```python
from build123d import *

# Parameters (mm, degrees)
SKETCH1_R           = 5
SKETCH1_R_2         = 1
BOSS_EXTRUDE1_DEPTH = 3
SKETCH2_R           = 8
BOSS_EXTRUDE2_DEPTH = 4
SKETCH4_R           = 1
CUT_EXTRUDE2_DEPTH  = 8
SKETCH3_RX          = 5.25
SKETCH3_RY          = 3.5
CUT_EXTRUDE1_DEPTH  = 2
SKETCH10_R          = 1
CUT_EXTRUDE5_DEPTH  = 7
SKETCH9_R           = 1.55
CUT_EXTRUDE4_DEPTH  = 3.5
CUT_EXTRUDE9_DEPTH  = 10
FILLET3_R           = 1
FILLET1_R           = 0.4


with BuildPart() as part:
    # Sketch1 → Boss-Extrude1 (new body)
    with BuildSketch(Plane.XY):
        Circle(SKETCH1_R)
        Circle(SKETCH1_R_2, mode=Mode.SUBTRACT)
    extrude(amount=BOSS_EXTRUDE1_DEPTH)

    # Sketch2 → Boss-Extrude2 (add)
    with BuildSketch(Plane.XY.offset(3)):
        Circle(SKETCH2_R)
    extrude(amount=BOSS_EXTRUDE2_DEPTH)

    # Sketch4 → Cut-Extrude2 (cut)
    with BuildSketch(Plane(origin=(0, 0, 3), x_dir=(-1, 0, 0), z_dir=(0, 0, -1))):
        with Locations(Location((0, 0, 0), (0, 0, 180))):
            Circle(SKETCH4_R)
    extrude(amount=-CUT_EXTRUDE2_DEPTH, mode=Mode.SUBTRACT)

    # Sketch3 → Cut-Extrude1 (cut)
    with BuildSketch(Plane.XY.offset(7)):
        with Locations(Location((0, 0), (0, 0, -90))):
            Ellipse(SKETCH3_RX, SKETCH3_RY)
    extrude(amount=-CUT_EXTRUDE1_DEPTH, mode=Mode.SUBTRACT)

    # Sketch10 → Cut-Extrude5 (cut)
    with BuildSketch(Plane(origin=(0, 0, 0), x_dir=(-1, 0, 0), z_dir=(0, 0, -1))):
        with BuildLine():
            Line((-2.25, -1.58113883), (-2.25, -3.605551275))
            ThreePointArc((-2.25, -3.605551275), (0, -4.25), (2.25, -3.605551275))
            Line((2.25, -3.605551275), (2.25, -1.58113883))
            ThreePointArc((2.25, -1.58113883), (0, 2.75), (-2.25, -1.58113883))
        make_face()
        Circle(SKETCH10_R, mode=Mode.SUBTRACT)
    extrude(amount=-CUT_EXTRUDE5_DEPTH, mode=Mode.SUBTRACT)

    # Sketch9 → Cut-Extrude4 (cut)
    with BuildSketch(Plane.XY.offset(7)):
        with Locations((-5.75, 0)):
            Circle(SKETCH9_R)
        with Locations((5.75, 0)):
            Circle(SKETCH9_R)
    extrude(amount=-CUT_EXTRUDE4_DEPTH, mode=Mode.SUBTRACT)

    # Sketch14 → Cut-Extrude9 (cut)
    with BuildSketch(Plane.XY.offset(5)):
        with BuildLine():
            Line((-2.4, -3.687817783), (-2.4, -1.62788206))
            ThreePointArc((-2.4, -1.62788206), (0, 2.9), (2.4, -1.62788206))
            Line((2.4, -1.62788206), (2.4, -3.687817783))
            ThreePointArc((2.4, -3.687817783), (0, -4.4), (-2.4, -3.687817783))
        make_face()
        with BuildLine():
            Line((2.25, -3.605551275), (2.25, -1.58113883))
            ThreePointArc((2.25, -1.58113883), (0, 2.75), (-2.25, -1.58113883))
            Line((-2.25, -1.58113883), (-2.25, -3.605551275))
            ThreePointArc((-2.25, -3.605551275), (0, -4.25), (2.25, -3.605551275))
        make_face(mode=Mode.SUBTRACT)
    extrude(amount=-CUT_EXTRUDE9_DEPTH, mode=Mode.SUBTRACT)

    # Fillet3
    fillet3_edges = [part.edges().sort_by_distance(p)[0] for p in [
        (2.4, -3.687817783, 2.5),
        (-2.4, -3.687817783, 2.5),
    ]]
    fillet(fillet3_edges, radius=FILLET3_R)

    # Fillet1
    fillet1_edges = [part.edges().sort_by_distance(p)[0] for p in [
        (-7.3, 0, 7),
        (4.2, 0, 7),
    ]]
    fillet(fillet1_edges, radius=FILLET1_R)


solid = part.part
```
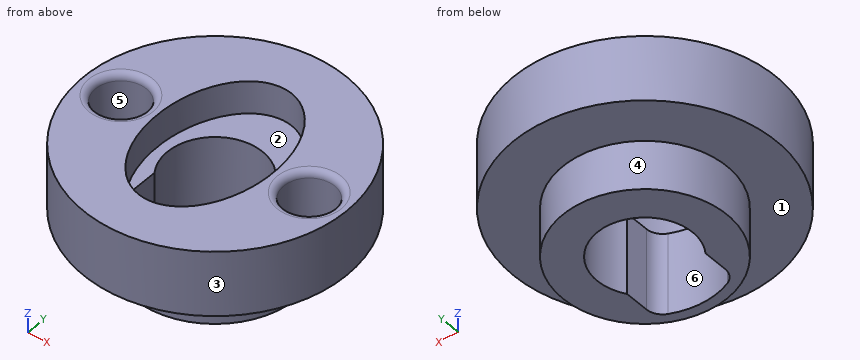
The model under review builds one solid part; all positions refer to its coordinate system, in mm. Face numbers are marked on the shaded views. A direction names the side the tool comes from. Round coordinates to 2 decimals unless told otherwise and drop trailing zeros. Order: outer loops, then holes, each group sorted by start corner. A loop starts at its lowest first (then second) coordinate and runs counter-clockwise, first axis right, second up.
Item 1: Add section C-C, the plane x = 5.75. State the section outline as (y, z) points.
Working result:
outline: (-5.56, 3) - (5.56, 3) - (5.56, 7) - (1.95, 7) arc R0.4 ccw to (1.55, 6.6) - (1.55, 3.5) - (-1.55, 3.5) - (-1.55, 6.6) arc R0.4 ccw to (-1.95, 7) - (-5.56, 7) - close
Item 2: Add section A-A, the plane z = 1.25. State the section outline as (x, y) points, and give its area (3 significant figures).
Working result:
outline: circle Ø10 at (0, 0); hole (-2.4, -3.1) arc R1 ccw to (-1.81, -4.01) arc R4.4 ccw to (1.81, -4.01) arc R1 ccw to (2.4, -3.1) - (2.4, -1.63) arc R2.9 ccw (long way) to (-2.4, -1.63) - close
area: 44.3 mm2
Item 3: To check wall thickness, follow probe 1 along Y at (x, z) = (0, 1.3); probe 2 along X at (y, z) = (-1, 4.75); probe 3 along Y at (x, z) = (0, 3.8). State the ranges of each line that lie inside material, in increasing order.
Working result:
probe 1: y = -5 to -4.4, 2.9 to 5
probe 2: x = -7.94 to -6.93, -4.57 to -2.72, 2.72 to 4.57, 6.93 to 7.94
probe 3: y = -8 to -4.4, 2.9 to 8
Item 4: Draft analysis for pull direction X (two halves, no side actions). For the marked faces 1, 2 and 3, state which applies: released by +X, released by -X, zero draft, split by the parting line, or undercut.
Working result:
face 1: zero draft
face 2: undercut
face 3: split by the parting line
Item 5: For pin 1 (1 mm diameter, centred on x = 5, z = 5, fed in from +Y); pin 2 (3.5 mm diameter, centred on x = -5.75, y = 0, fed in from +Z); pin 3 (0.7 mm diameter, centred on y = -2.5, z = 3.5, fed in from +X); pin 4 (3.5 mm diameter, centred on x = 0, y = 0, fed in from +Z), all flat-tipped, find the tip position at first contact; note any pin that passes through.
Working result:
pin 1: stops at y = 6.61
pin 2: stops at z = 6.95
pin 3: stops at x = 7.71
pin 4: passes through
Item 6: Machinability: for the marked faces 4, 5 and 6, which of the approach directions +Z, -Z, +X, -X, +Y, -Y give a long, thin tool a straight path to every point of the face, cutting with its end or side? Answer none if there is none.
Working result:
face 4: -Z
face 5: +Z
face 6: +Z, -Z
Item 7: Add section B-B, the plane z = 4.75. State the section outline as (x, y) points, and give its area (3 significant figures).
Working result:
outline: circle Ø16 at (0, 0); hole circle Ø3.1 at (-5.75, 0); hole (-2.4, -3.1) arc R1 ccw to (-1.81, -4.01) arc R4.4 ccw to (1.81, -4.01) arc R1 ccw to (2.4, -3.1) - (2.4, -1.63) arc R2.9 ccw (long way) to (-2.4, -1.63) - close; hole circle Ø3.1 at (5.75, 0)
area: 152 mm2
Item 8: Add section D-D, the plane y = 5.5. State the section outline as (x, z) points, and give its area (3 significant figures).
Working result:
outline: (-5.81, 3) - (5.81, 3) - (5.81, 7) - (-5.81, 7) - close
area: 46.5 mm2
